Can you work these out from the model? Positions are in its coordinate system, mm. A direction names the side the tool comes from. Coordinates: 2 decimals unless noted, no trailing zeros. Order: outer loops, then holes, each group sorted by start corner. A loop starts at its lowest first (then second) coordinate and runs counter-clockwise, first axis right, second up. Notation, with made-up numbers: (66.25, 49.5) - (86.25, 49.5) arc R36 cw to (86.25, 86.5) - close; hole circle Ø3 at (4, -10). An arc over 180 degrees is marked (long way). Return JSON: item names as keys, results as strings. Group by question number.
1) Imagine slicing it at A-A (z = -7.5). Give the number of separate pieces and of enclosed holes in the cut face, and give its area (3 significant figures).
2) Imagine slicing it at B-B (y = 19). Write out the boundary of the cut face in (x, z).
3) Imagine slicing it at C-C (x = -9). Write out the boundary of the cut face in (y, z).
4) If I drill on line 1 along X through (y, z) = (29, 0); line 2 along X through (y, z) = (9.5, -2.5); line 3 along Y through (x, z) = (-2, 2), over which ranges is the centre line in solid material (lowest first)?
5) Which directions (+Z, -Z, +X, -X, +Y, -Y) give clear straight access to the entire face, cutting with the end or side of a thin tool? Please do faces 4 (the face through (-33, 5, 0)), 5 (the face through (-2, 0, 0)).
6) If we mould it in two halves opening along Z, with no side actions, what happens to faces 1 (the face through (1, 1, -1)), 2 (the face through (34.316, 22.252, -0.337)), 3 (the face through (28, 5, 0))? For each: pulls with the +Z half, pulls with the -Z half, needs draft (parallel to the pull), parting line crosses it, or undercut.
7) For pin 1 Ø1.1 at (y, z) = (0.5, -5) entering from -X; pin 2 Ø0.5 at (y, z) = (0.5, -2.5) entering from -X; pin 3 Ø1.1 at (y, z) = (0.5, -4) entering from -X, each with a flat end and sliding along its axis, tell me the tip position at first contact or that it passes through.
```python
from build123d import *

# Parameters (mm, degrees)
BOSS_EXTRUDE1_DEPTH = 1
SKETCH5_R           = 4
CUT_EXTRUDE1_DEPTH  = 35


with BuildPart() as part:
    # Sketch2 → Boss-Extrude1 (new body)
    with BuildSketch(Plane(origin=(0, 0, 0), x_dir=(1, 0, 0), z_dir=(0, 1, 0))):
        with BuildLine():
            Line((-32.760220782, -0.5), (-23.260220782, -0.5))
            ThreePointArc((-23.260220782, -0.5), (-22.553114001, -0.207106781), (-22.260220782, 0.5))
            Line((-22.260220782, 0.5), (-22.260220782, 14.5))
            Line((-22.260220782, 14.5), (-20.260220782, 14.5))
            Line((-20.260220782, 14.5), (-20.260220782, 0))
            Line((-20.260220782, 0), (-20.260220782, -14.5))
            ThreePointArc((-20.260220782, -14.5), (-19.967327563, -15.207106781), (-19.260220782, -15.5))
            Line((-19.260220782, -15.5), (-17.260220782, -15.5))
            ThreePointArc((-17.260220782, -15.5), (-16.553114001, -15.207106781), (-16.260220782, -14.5))
            Line((-16.260220782, -14.5), (-16.260220782, 0))
            Line((-16.260220782, 0), (-16.260220782, 14.5))
            Line((-16.260220782, 14.5), (-14.174535805, 14.5))
            Line((-14.174535805, 14.5), (-14.174535805, -14.5))
            ThreePointArc((-14.174535805, -14.5), (-13.881642586, -15.207106781), (-13.174535805, -15.5))
            Line((-13.174535805, -15.5), (-11.174535805, -15.5))
            ThreePointArc((-11.174535805, -15.5), (-10.467429024, -15.207106781), (-10.174535805, -14.5))
            Line((-10.174535805, -14.5), (-10.174535805, 14.5))
            Line((-10.174535805, 14.5), (-8.174535805, 14.5))
            Line((-8.174535805, 14.5), (-8.174535805, -14.5))
            ThreePointArc((-8.174535805, -14.5), (-7.881642586, -15.207106781), (-7.174535805, -15.5))
            Line((-7.174535805, -15.5), (-5.174535805, -15.5))
            ThreePointArc((-5.174535805, -15.5), (-4.467429024, -15.207106781), (-4.174535805, -14.5))
            Line((-4.174535805, -14.5), (-4.174535805, 14.5))
            Line((-4.174535805, 14.5), (-2.174535805, 14.5))
            Line((-2.174535805, 14.5), (-2.174535805, -14.5))
            ThreePointArc((-2.174535805, -14.5), (-1.881642586, -15.207106781), (-1.174535805, -15.5))
            Line((-1.174535805, -15.5), (0.825464195, -15.5))
            ThreePointArc((0.825464195, -15.5), (1.532570976, -15.207106781), (1.825464195, -14.5))
            Line((1.825464195, -14.5), (1.825464195, 14.5))
            Line((1.825464195, 14.5), (3.825464195, 14.5))
            Line((3.825464195, 14.5), (3.825464195, -14.5))
            ThreePointArc((3.825464195, -14.5), (4.118357414, -15.207106781), (4.825464195, -15.5))
            Line((4.825464195, -15.5), (6.825464195, -15.5))
            ThreePointArc((6.825464195, -15.5), (7.532570976, -15.207106781), (7.825464195, -14.5))
            Line((7.825464195, -14.5), (7.825464195, 14.5))
            Line((7.825464195, 14.5), (9.825464195, 14.5))
            Line((9.825464195, 14.5), (9.825464195, -14.5))
            ThreePointArc((9.825464195, -14.5), (10.118357414, -15.207106781), (10.825464195, -15.5))
            Line((10.825464195, -15.5), (12.825464195, -15.5))
            ThreePointArc((12.825464195, -15.5), (13.532570976, -15.207106781), (13.825464195, -14.5))
            Line((13.825464195, -14.5), (13.825464195, -0.5))
            Line((13.825464195, -0.5), (28.325464195, -0.5))
            ThreePointArc((28.325464195, -0.5), (28.825464195, 0), (28.325464195, 0.5))
            Line((28.325464195, 0.5), (13.825464195, 0.5))
            ThreePointArc((13.825464195, 0.5), (13.118357414, 0.207106781), (12.825464195, -0.5))
            Line((12.825464195, -0.5), (12.825464195, -14.5))
            Line((12.825464195, -14.5), (10.825464195, -14.5))
            Line((10.825464195, -14.5), (10.825464195, 14.5))
            ThreePointArc((10.825464195, 14.5), (10.532570976, 15.207106781), (9.825464195, 15.5))
            Line((9.825464195, 15.5), (7.825464195, 15.5))
            ThreePointArc((7.825464195, 15.5), (7.118357414, 15.207106781), (6.825464195, 14.5))
            Line((6.825464195, 14.5), (6.825464195, -14.5))
            Line((6.825464195, -14.5), (4.825464195, -14.5))
            Line((4.825464195, -14.5), (4.825464195, 14.5))
            ThreePointArc((4.825464195, 14.5), (4.532570976, 15.207106781), (3.825464195, 15.5))
            Line((3.825464195, 15.5), (1.825464195, 15.5))
            ThreePointArc((1.825464195, 15.5), (1.118357414, 15.207106781), (0.825464195, 14.5))
            Line((0.825464195, 14.5), (0.825464195, -14.5))
            Line((0.825464195, -14.5), (-1.174535805, -14.5))
            Line((-1.174535805, -14.5), (-1.174535805, 14.5))
            ThreePointArc((-1.174535805, 14.5), (-1.467429024, 15.207106781), (-2.174535805, 15.5))
            Line((-2.174535805, 15.5), (-4.174535805, 15.5))
            ThreePointArc((-4.174535805, 15.5), (-4.881642586, 15.207106781), (-5.174535805, 14.5))
            Line((-5.174535805, 14.5), (-5.174535805, -14.5))
            Line((-5.174535805, -14.5), (-7.174535805, -14.5))
            Line((-7.174535805, -14.5), (-7.174535805, 14.5))
            ThreePointArc((-7.174535805, 14.5), (-7.467429024, 15.207106781), (-8.174535805, 15.5))
            Line((-8.174535805, 15.5), (-10.174535805, 15.5))
            ThreePointArc((-10.174535805, 15.5), (-10.881642586, 15.207106781), (-11.174535805, 14.5))
            Line((-11.174535805, 14.5), (-11.174535805, -14.5))
            Line((-11.174535805, -14.5), (-13.174535805, -14.5))
            Line((-13.174535805, -14.5), (-13.174535805, 14.5))
            ThreePointArc((-13.174535805, 14.5), (-13.467429024, 15.207106781), (-14.174535805, 15.5))
            Line((-14.174535805, 15.5), (-16.260220782, 15.5))
            ThreePointArc((-16.260220782, 15.5), (-16.967327563, 15.207106781), (-17.260220782, 14.5))
            Line((-17.260220782, 14.5), (-17.260220782, 0))
            Line((-17.260220782, 0), (-17.260220782, -14.5))
            Line((-17.260220782, -14.5), (-19.260220782, -14.5))
            Line((-19.260220782, -14.5), (-19.260220782, 0))
            Line((-19.260220782, 0), (-19.260220782, 14.5))
            ThreePointArc((-19.260220782, 14.5), (-19.553114001, 15.207106781), (-20.260220782, 15.5))
            Line((-20.260220782, 15.5), (-22.260220782, 15.5))
            ThreePointArc((-22.260220782, 15.5), (-22.967327563, 15.207106781), (-23.260220782, 14.5))
            Line((-23.260220782, 14.5), (-23.260220782, 0.5))
            Line((-23.260220782, 0.5), (-32.760220782, 0.5))
            ThreePointArc((-32.760220782, 0.5), (-33.260220782, 0), (-32.760220782, -0.5))
        make_face()
    extrude(amount=BOSS_EXTRUDE1_DEPTH)

    # Sketch3 → Revolve1 (revolve)
    with BuildSketch(Plane.XY, mode=Mode.PRIVATE) as revolve1_sk:
        Polygon((-32.760220782, 0), (-37.760220782, 0), (-38.760220782, 4), (-38.760220782, 40), (-32.760220782, 40), align=None)
    revolve(revolve1_sk.sketch.rotate(Axis((-32.760220782, 0, 0), (0, 1, 0)), 174.260829523), axis=Axis((-32.760220782, 0, 0), (0, 1, 0)))

    # Sketch4 → Revolve2 (revolve)
    with BuildSketch(Plane.XY, mode=Mode.PRIVATE) as revolve2_sk:
        Polygon((28.325464195, 0), (33.325464195, 0), (34.325464195, 4), (34.325464195, 40), (28.325464195, 40), align=None)
    revolve(revolve2_sk.sketch.rotate(Axis((28.325464195, 0, 0), (0, 1, 0)), 185.739170027), axis=Axis((28.325464195, 0, 0), (0, 1, 0)))

    # Sketch5 → Cut-Extrude1 (cut)
    with BuildSketch(Plane(origin=(0, 40, 0), x_dir=(1, 0, 0), z_dir=(0, 1, 0))):
        with Locations(Location((-32.760220782, 0, 0), (0, 0, 270))):
            Circle(SKETCH5_R)
        with Locations(Location((28.325464195, 0, 0), (0, 0, 270))):
            Circle(SKETCH5_R)
    extrude(amount=-CUT_EXTRUDE1_DEPTH, mode=Mode.SUBTRACT)


solid = part.part
```
Calculated:
{
 "1": {"separate pieces": "12", "enclosed holes": "0", "area": "12.0 mm2"},
 "2": {"outline": "circle Ø12 at (-32.76, 0); circle Ø12 at (28.33, 0); hole circle Ø8 at (-32.76, 0); hole circle Ø8 at (28.33, 0)"},
 "3": {"outline": "(0, -15.5) - (1, -15.5) - (1, -14.5) - (0, -14.5) - close"},
 "4": {"line 1": "-38.76 to -36.76, -28.76 to -26.76, 22.33 to 24.33, 32.33 to 34.33", "line 2": "-38.21 to -35.88, -29.64 to -27.31, 22.87 to 25.2, 31.45 to 33.78", "line 3": "0 to 1"},
 "5": {"face 4": "+Y", "face 5": "+Z, -Z, +X, -X, -Y"},
 "6": {"face 1": "needs draft", "face 2": "parting line crosses it", "face 3": "undercut"},
 "7": {"pin 1": "x = -35.34", "pin 2": "x = -37.38", "pin 3": "x = -36.58"}
}
